from build123d import *

# Parameters (mm, degrees)
SKETCH_1_W      = 60
SKETCH_1_H      = 2
EXTRUDE_1_DEPTH = 40
SKETCH_3_R      = 1.55
EXTRUDE_2_DEPTH = 2
EXTRUDE_3_DEPTH = 60


with BuildPart() as part:
    # Sketch 1 → Extrude 1 (new body)
    with BuildSketch(Plane(origin=(0, 0, 0), x_dir=(1, 0, 0), z_dir=(0, 1, 0))):
        Rectangle(SKETCH_1_W, SKETCH_1_H)
    extrude(amount=EXTRUDE_1_DEPTH)



with BuildPart() as body_2:
    # Sketch 3 → Extrude 2 (new, through all)
    with BuildSketch(Plane(origin=(0, 0, -1), x_dir=(-1, 0, 0), z_dir=(0, 0, -1))):
        with BuildLine():
            Line((-7.994757435, 0), (-4.05536846, -6.823221856))
            ThreePointArc((-4.05536846, -6.823221856), (-0.01683957, -9.154867598), (4.02168932, -6.823221856))
            Line((4.02168932, -6.823221856), (7.961078295, 0))
            Line((7.961078295, 0), (-7.994757435, 0))
        make_face()
        with Locations((-0.01683957, -4.491576114)):
            Circle(SKETCH_3_R, mode=Mode.SUBTRACT)
    extrude(amount=-EXTRUDE_2_DEPTH)


with BuildPart() as part_1:
    add(part.part)

    add(body_2.part)  # Extrude 3 merges body 2
    # Sketch 4 → Extrude 3 (add, through all)
    with BuildSketch(Plane(origin=(30, 0, 0), x_dir=(0, 0, -1), z_dir=(1, 0, 0))):
        with BuildLine():
            Line((5, 36), (5, -1.993440082))
            Line((5, -1.993440082), (3, -1.993440082))
            Line((3, -1.993440082), (3, 33.134423916))
            ThreePointArc((3, 33.134423916), (2.461049161, 35.065394885), (1, 36.43814841))
            Line((1, 36.43814841), (1, 40))
            ThreePointArc((1, 40), (3.828427125, 38.828427125), (5, 36))
        make_face()
        with BuildLine():
            Line((-5, 36), (-5, -1.993440082))
            Line((-5, -1.993440082), (-3, -1.993440082))
            Line((-3, -1.993440082), (-3, 33.134423916))
            ThreePointArc((-3, 33.134423916), (-2.461049161, 35.065394885), (-1, 36.43814841))
            Line((-1, 36.43814841), (-1, 40))
            ThreePointArc((-1, 40), (-3.828427125, 38.828427125), (-5, 36))
        make_face()
    extrude(amount=-EXTRUDE_3_DEPTH)


solid = part_1.part
Geometry: final body of the model. Coordinates: model frame, mm. A direction names the side the tool comes from. Give positions to 0.01 mm unless a question says otherwise; leave off trailing zeros. Loops run counter-clockwise (first coordinate to the right, second up) from the corner with the lowest first, then second, coordinate; pieces in that order, holes last. Notation, with made-up numbers: M 79,59 L 119,59 A15 ccw 119,65 Z; hole C 44.5,68.25 d2. An arc over 180 degrees is marked long. Put each result on its own line as item: value. Start each with the question number.
1) Pull-direction query (Z, two-part tool) for faces 4 (the flat face through (0, 15, -3)), 5 (the cylindrical face through (0.085, -9.154, -0.014)), 6 (the flat face through (0, 17, -5)); classes: pulls with the +Z half, pulls with the -Z half, needs draft (parallel to the pull), parting line crosses it, or undercut.
2) Ray query, line 1 along Z through (x, y) = (23, 19); line 2 along Z through (x, y) = (-6, 35.5); line 3 along Y through (x, z) = (-25.5, -0.5). Return the intervals inside material, ascending.
3) Cut plane A-A (y = 4.5). Output: boundary loops of the cut face in (x, z), then the cut area to 3 significant figures.
4) Contact query for flat-ended pins moving along their axis: pin 1 (2.5 mm diameter, centred on x = 0.02, y = -4.49, fed in from -Z); pin 2 (1.6 mm diameter, centred on x = -24.5, z = 0, fed in from -Y); pin 3 (3 mm diameter, centred on y = 2, z = 2.5, fed in from +X); pin 4 (3 mm diameter, centred on x = 20, z = 2, fed in from -Y). Output: stop coordinate, or through.
5) Cut plane B-B (x = -9). Output: boundary loops of the cut face in (y, z), then the cut area to 3 significant figures.
6) Cut plane C-C (z = 2.25). Output: boundary loops of the cut face in (x, y), then the cut area to 3 significant figures.
7) Access query for faces 1 (the flat face through (-5.964, -3.459, -0.014)), 2 (the flat face through (0, -1.993, -4)), 3 (the flat face through (0, 18, 1)). Directions: +Z, -Z, +X, -X, +Y, -Y. A direction counts if a zero-diameter tool reaches every point of the face in a straight line with its end or side. Return the directions, or none.
Verdict:
1. face 4: undercut
1. face 5: needs draft
1. face 6: pulls with the -Z half
2. line 1: -5 to -3, -1 to 1, 3 to 5
2. line 2: -5 to -2.15, -1 to 1, 2.15 to 5
2. line 3: 0 to 40
3. outline: M -30,-5 L 30,-5 L 30,-3 L -30,-3 Z; M -30,-1 L 30,-1 L 30,1 L -30,1 Z; M -30,3 L 30,3 L 30,5 L -30,5 Z
3. area: 360 mm2
4. pin 1: through
4. pin 2: y = 0
4. pin 3: x = 30
4. pin 4: y = -1.99
5. outline: M -1.99,-5 L 36,-5 A4 ccw 40,-1 L 40,1 A4 ccw 36,5 L -1.99,5 L -1.99,3 L 33.13,3 A3.73 cw 36.44,1 L 0,1 L 0,-1 L 36.44,-1 A3.73 cw 33.13,-3 L -1.99,-3 Z
5. area: 259 mm2
6. outline: M -30,35.38 L 30,35.38 L 30,39.8 L -30,39.8 Z
6. area: 265 mm2
7. face 1: -X, -Y
7. face 2: -Z, +X, -X, -Y
7. face 3: +X, -X, -Y
